from build123d import *

# Parameters (mm, degrees)
SKETCH1_W           = 20
SKETCH1_H           = 28
BOSS_EXTRUDE1_DEPTH = 4
SKETCH2_R           = 1.7
CUT_EXTRUDE1_DEPTH  = 4
SKETCH6_W           = 40
SKETCH6_H           = 28
BOSS_EXTRUDE2_DEPTH = 4
SKETCH7_W           = 2
SKETCH7_H           = 28
BOSS_EXTRUDE3_DEPTH = 4
CHAMFER2_SIZE       = 1
SKETCH8_R           = 2.15
SKETCH8_R_2         = 1.5
CUT_EXTRUDE2_DEPTH  = 4
SKETCH12_W          = 62
SKETCH12_H          = 4
BOSS_EXTRUDE4_DEPTH = 1
SKETCH13_W          = 62
SKETCH13_H          = 4
BOSS_EXTRUDE5_DEPTH = 1


with BuildPart() as part:
    # Sketch1 → Boss-Extrude1 (new body)
    with BuildSketch(Plane(origin=(0, 0, 0), x_dir=(1, 0, 0), z_dir=(0, 1, 0))):
        Rectangle(SKETCH1_W, SKETCH1_H)
    extrude(amount=BOSS_EXTRUDE1_DEPTH)

    # Sketch2 → Cut-Extrude1 (cut)
    with BuildSketch(Plane(origin=(0, 4, 0), x_dir=(1, 0, 0), z_dir=(0, 1, 0))):
        with Locations(Location((-7.5, 5, 0), (0, 0, 270))):
            Circle(SKETCH2_R)
        with Locations(Location((-7.5, -5, 0), (0, 0, 270))):
            Circle(SKETCH2_R)
        with Locations(Location((7.5, -5, 0), (0, 0, 270))):
            Circle(SKETCH2_R)
        with Locations(Location((7.5, 5, 0), (0, 0, 270))):
            Circle(SKETCH2_R)
    extrude(amount=-CUT_EXTRUDE1_DEPTH, mode=Mode.SUBTRACT)

    # Sketch6 → Boss-Extrude2 (add)
    with BuildSketch(Plane(origin=(0, 4, 0), x_dir=(1, 0, 0), z_dir=(0, 1, 0))):
        with Locations((30, 0)):
            Rectangle(SKETCH6_W, SKETCH6_H)
    extrude(amount=-BOSS_EXTRUDE2_DEPTH)

    # Sketch7 → Boss-Extrude3 (add)
    with BuildSketch(Plane(origin=(0, 4, 0), x_dir=(1, 0, 0), z_dir=(0, 1, 0))):
        with Locations((-11, 0)):
            Rectangle(SKETCH7_W, SKETCH7_H)
    extrude(amount=-BOSS_EXTRUDE3_DEPTH)

    # Chamfer2
    chamfer2_edges = [part.edges().sort_by_distance(p)[0] for p in [
        (-7.5, 4, 3.3),
        (7.5, 4, -6.7),
        (-7.5, 4, -6.7),
        (7.5, 4, 3.3),
    ]]
    chamfer(chamfer2_edges, length=CHAMFER2_SIZE)

    # Sketch8 → Cut-Extrude2 (cut)
    with BuildSketch(Plane(origin=(0, 4, 0), x_dir=(1, 0, 0), z_dir=(0, 1, 0))):
        with Locations(Location((34.703187254, 0, 0), (0, 0, 270))):
            Circle(SKETCH8_R)
        with Locations(Location((29.203187254, 5.5, 0), (0, 0, 270))):
            Circle(SKETCH8_R_2)
        with Locations(Location((40.203187254, 5.5, 0), (0, 0, 270))):
            Circle(SKETCH8_R_2)
        with Locations(Location((40.203187254, -5.5, 0), (0, 0, 270))):
            Circle(SKETCH8_R_2)
        with Locations(Location((29.203187254, -5.5, 0), (0, 0, 270))):
            Circle(SKETCH8_R_2)
    extrude(amount=-CUT_EXTRUDE2_DEPTH, mode=Mode.SUBTRACT)

    # Sketch12 → Boss-Extrude4 (add)
    with BuildSketch(Plane.XY.offset(14)):
        with Locations((19, 2)):
            Rectangle(SKETCH12_W, SKETCH12_H)
    extrude(amount=BOSS_EXTRUDE4_DEPTH)

    # Sketch13 → Boss-Extrude5 (add)
    with BuildSketch(Plane(origin=(0, 0, -14), x_dir=(-1, 0, 0), z_dir=(0, 0, -1))):
        with Locations((-19, 2)):
            Rectangle(SKETCH13_W, SKETCH13_H)
    extrude(amount=BOSS_EXTRUDE5_DEPTH)


solid = part.part
Part model, mm, in its own coordinate system. Coordinates: 2 decimals unless noted, no trailing zeros. Order: outer loops, then holes, each group sorted by start corner. A loop starts at its lowest first (then second) coordinate and runs counter-clockwise, first axis right, second up. Notation, with made-up numbers: M 25.5,54.5 L 82.5,54.5 A20 cw 82.5,72.5 Z; hole C 59,-22 d4. An arc over 180 degrees is marked long. Use a Markdown table: item, result.
(1) Cut at A-A on z = 0. Write the cut outline in (x, y), then the cut area to 3 significant figures.
A:
| item | result |
|---|---|
| outline | M -12,0 L 32.55,0 L 32.55,4 L -12,4 Z; M 36.85,0 L 50,0 L 50,4 L 36.85,4 Z |
| area | 231 mm^2 |
(2) Probe L1, parallel to X at y = 1.25, z = -5; L2, parallel to Z at x = 29.5, y = 0.6; L3, parallel to X at y = 2.5, z = 5.75. List the from-to ranges inside material, lowest first.
A:
| item | result |
|---|---|
| L1 | x = -12 to -9.2, -5.8 to 5.8, 9.2 to 27.79, 30.62 to 38.79, 41.62 to 50 |
| L2 | z = -15 to -6.97, -4.03 to 4.03, 6.97 to 15 |
| L3 | x = -12 to -9.03, -5.97 to 5.97, 9.03 to 27.72, 30.68 to 38.72, 41.68 to 50 |
(3) Cut at B-B on x = 7.5. Write the cut outline in (y, z).
A:
| item | result |
|---|---|
| outline | M 0,-15 L 4,-15 L 4,-7.7 L 3,-6.7 L 0,-6.7 Z; M 0,-3.3 L 3,-3.3 L 4,-2.3 L 4,2.3 L 3,3.3 L 0,3.3 Z; M 0,6.7 L 3,6.7 L 4,7.7 L 4,15 L 0,15 Z |
(4) Cut at D-D on z = 5. Write the cut outline in (x, y).
A:
| item | result |
|---|---|
| outline | M -12,0 L -9.2,0 L -9.2,3 L -10.2,4 L -12,4 Z; M -5.8,0 L 5.8,0 L 5.8,3 L 4.8,4 L -4.8,4 L -5.8,3 Z; M 9.2,0 L 27.79,0 L 27.79,4 L 10.2,4 L 9.2,3 Z; M 30.62,0 L 38.79,0 L 38.79,4 L 30.62,4 Z; M 41.62,0 L 50,0 L 50,4 L 41.62,4 Z |
(5) Flat gauge pins, fed straight in: pin 1 (5.5 mm diameter, centred on x = -7.5, z = -5, fed in from -Y); pin 2 (4.5 mm diameter, centred on x = 7.5, z = -5, fed in from +Y). Where does each tip first touch, or does it go through?
A:
| item | result |
|---|---|
| pin 1 | stops at y = 0 |
| pin 2 | stops at y = 3.55 |
(6) Pull direction X, two halves, no side cores. Call faces 1 (the flat face through (50, 2, 0)), 2 (the cylindrical face through (32.604, 2.028, -0.466)), 3 (the flat face through (19, 0, 0)), 4 (the cylindrical face through (-9, 1.5, 5.8)): released by +X, released by -X, zero draft, split by the parting line, or undercut.
A:
| item | result |
|---|---|
| face 1 | released by +X |
| face 2 | undercut |
| face 3 | zero draft |
| face 4 | undercut |
(7) Cut at C-C on y = 1.1. State how many separate pieces and enclosed holes the cut face has, then the cut area to 3 significant figures.
A:
| item | result |
|---|---|
| separate pieces | 1 |
| enclosed holes | 9 |
| area | 1,780 mm^2 |
